Geometry: final body of the model. Coordinates: model frame, mm. A direction names the side the tool comes from. Give positions to 0.01 mm unless a question says otherwise; leave off trailing zeros. Loops run counter-clockwise (first coordinate to the right, second up) from the corner with the lowest first, then second, coordinate; pieces in that order, holes last.
1. Section D-D, the plane z = -7.5. Output: boundary loops of the cut face in (x, y), then the cut area to 3 significant figures.
2. Section A-A, the plane x = -18. Output: boundary loops of the cut face in (y, z).
3. Material intervals for line 1 along Z through (x, y) = (-3, 0.95); line 2 along X through (y, z) = (4.5, 1); line 3 along X through (y, z) = (3.25, -10), sorted ascending.
4. First-contact query: P1, Ø1, axis at x = -28.5, y = 1, coming from the -Z side; P2, Ø1.6, axis at x = -9, y = 1, coming from the +Z side; P3, Ø1, axis at y = 3.5, z = -6.5, coming from the +X side; P4, Ø4, axis at x = -18, z = -5, coming from the +Y side. Flat tips, straight axial feed; report the tip coordinate or a pass-through.
5. Section B-B, the plane z = -5. Output: boundary loops of the cut face in (x, y).
6. Access query for faces 5 (the face through (-6, 1, -10)), 6 (the face through (-30, 1, -10)), 7 (the face through (-30, 1, 0)). Directions: +Z, -Z, +X, -X, +Y, -Y. A direction counts if a zero-diameter tool reaches every point of the face in a straight line with its end or side. Return the directions, or none.
7. Draft query along X for faces 1 (the face through (-20, 7, -8)), 2 (the face through (-24.743, 3.451, -4.703)), 3 (the face through (-16, 9, -2)), 4 (the face through (-18.976, 4.563, -12.436)). Return one class per face: +X half, -X half, draft (parallel to the pull), parting line (faces both ways), or undercut.
8. Section C-C, the plane x = -33. Output: boundary loops of the cut face in (y, z).
Autodesk Inventor part; units mm, degrees
ref_plane "YZ Plane" through (0, 0, 0) normal (1, 0, 0) x (0, 1, 0)
ref_plane "XZ Plane" through (0, 0, 0) normal (0, 1, 0) x (-1, 0, 0)
ref_plane "XY Plane" through (0, 0, 0) normal (0, 0, 1) x (1, 0, 0)
sketch "Sketch1" plane through (0, 0, 0) normal (0, 1, 0) x (-1, 0, 0)
  line L0 (0, 0) -> (0, -10)
  line L1 (0, -10) -> (36, -10)
  line L2 (36, -10) -> (36, 0)
  line L3 (36, 0) -> (0, 0)
  circle A0 centre (33, -5) radius 1.5
  circle A1 centre (3, -5) radius 1.5
  dimension "d0" = 10
  dimension "d1" = 36
extrude "Extrusion1" add sketch "Sketch1" along normal blind 2
sketch "Sketch2" plane through (0, 2, 0) normal (0, 1, 0) x (1, 0, 0)
  line L0 (-36, 0) -> (0, 0)
  line L1 (-18, 0) -> (-18, 10)
  line L2 (0, 10) -> (-36, 10)
  circle A0 centre (-18, 5) radius 7.5
  dimension "d6" = 15
extrude "Extrusion2" add sketch "Sketch2" along normal blind 7
sketch "Sketch5" plane through (0, 2, 0) normal (0, -1, 0) x (1, 0, 0)
  arc A0 (-13.4654, 0) -> (-22.5346, 0) centre (-18, -5) ccw
  circle A1 centre (-18, -5) radius 7.5
  point P0 (0, 0)
extrude "Extrusion5" add sketch "Sketch5" along normal blind 2
sketch "Sketch8" plane through (-18, 9, -5) normal (0, 1, 0) x (1, 0, 0)
  circle A0 centre (0, 0) radius 3.25
  point P0 (18, -5)
  dimension "d19" = 6.5
extrude "Extrusion7" cut sketch "Sketch8" against normal up to next
sketch "Sketch9" plane through (0, 0, 0) normal (0, -1, 0) x (1, 0, 0)
  circle A0 centre (-18, -5) radius 3.25
  circle A1 centre (-18, -5) radius 6.75
  point P0 (0, 0)
  dimension "d22" = 13.5
extrude "Extrusion8" cut sketch "Sketch9" against normal blind 7
properties part number "LED_mount2"
Answers below:
1. outline: (-36, 0) - (-24.27, 0) - (-24.27, 7) - (-20.08, 7) - (-20.08, 9) - (-25.07, 9) - (-25.07, 2) - (-36, 2) - close; (-15.92, 7) - (-11.73, 7) - (-11.73, 0) - (0, 0) - (0, 2) - (-10.93, 2) - (-10.93, 9) - (-15.92, 9) - close
1. area: 74.9 mm2
2. outline: (0, -12.5) - (9, -12.5) - (9, -8.25) - (7, -8.25) - (7, -11.75) - (0, -11.75) - close; (0, 1.75) - (7, 1.75) - (7, -1.75) - (9, -1.75) - (9, 2.5) - (0, 2.5) - close
3. line 1: z = -10 to -6.5, -3.5 to 0
3. line 2: x = -22.5 to -21.09, -14.91 to -13.5
3. line 3: x = -23.59 to -22.53, -13.47 to -12.41
4. P1: stops at z = -10
4. P2: stops at z = 0
4. P3: stops at x = -10.57
4. P4: passes through
5. outline: (-36, 0) - (-34.5, 0) - (-34.5, 2) - (-36, 2) - close; (-31.5, 0) - (-24.75, 0) - (-24.75, 7) - (-21.25, 7) - (-21.25, 9) - (-25.5, 9) - (-25.5, 2) - (-31.5, 2) - close; (-14.75, 7) - (-11.25, 7) - (-11.25, 0) - (-4.5, 0) - (-4.5, 2) - (-10.5, 2) - (-10.5, 9) - (-14.75, 9) - close; (-1.5, 0) - (0, 0) - (0, 2) - (-1.5, 2) - close
6. face 5: -Z, +X, +Y, -Y
6. face 6: -Z, -X, +Y, -Y
6. face 7: +Z, -X, +Y, -Y
7. face 1: undercut
7. face 2: undercut
7. face 3: draft
7. face 4: parting line
8. outline: (0, -10) - (2, -10) - (2, -6.5) - (0, -6.5) - close; (0, -3.5) - (2, -3.5) - (2, 0) - (0, 0) - close
